CAD build for the part. Positions are in the model's coordinates, mm. Face numbers are marked on the shaded views. A direction names the side the tool comes from. Round coordinates to 2 decimals unless told otherwise and drop trailing zeros. Order: outer loops, then holes, each group sorted by start corner. A loop starts at its lowest first (then second) coordinate and runs counter-clockwise, first axis right, second up.
```python
from build123d import *

# Parameters (mm, degrees)
BOSS_EXTRUDE1_DEPTH = 101.6


with BuildPart() as part:
    # Sketch1 → Boss-Extrude1 (new body)
    with BuildSketch(Plane.XY):
        with BuildLine():
            Line((-101.6, -5178.34108), (-101.6, -5168.81608))
            Line((-101.6, -5168.81608), (-190.441035714, -5168.81608))
            Line((-190.441035714, -5168.81608), (-190.441035714, -5175.16608))
            ThreePointArc((-190.441035714, -5175.16608), (-189.511099745, -5177.41114403), (-187.266035714, -5178.34108))
            Line((-187.266035714, -5178.34108), (-101.6, -5178.34108))
        make_face()
        with BuildLine():
            Line((-38.041035714, -5168.81608), (-47.566035714, -5168.81608))
            Line((-47.566035714, -5168.81608), (-53.408035714, -5168.81608))
            Line((-53.408035714, -5168.81608), (-101.6, -5168.81608))
            Line((-101.6, -5168.81608), (-101.6, -5178.34108))
            Line((-101.6, -5178.34108), (-41.216035714, -5178.34108))
            ThreePointArc((-41.216035714, -5178.34108), (-38.970971684, -5177.41114403), (-38.041035714, -5175.16608))
            Line((-38.041035714, -5175.16608), (-38.041035714, -5168.81608))
        make_face()
        with BuildLine():
            Line((-47.566035714, -5025.94108), (-47.566035714, -5168.81608))
            Line((-47.566035714, -5168.81608), (-38.041035714, -5168.81608))
            Line((-38.041035714, -5168.81608), (-38.041035714, -5029.11608))
            ThreePointArc((-38.041035714, -5029.11608), (-38.970971684, -5026.87101597), (-41.216035714, -5025.94108))
            Line((-41.216035714, -5025.94108), (-47.566035714, -5025.94108))
        make_face()
    extrude(amount=-BOSS_EXTRUDE1_DEPTH)


solid = part.part
```
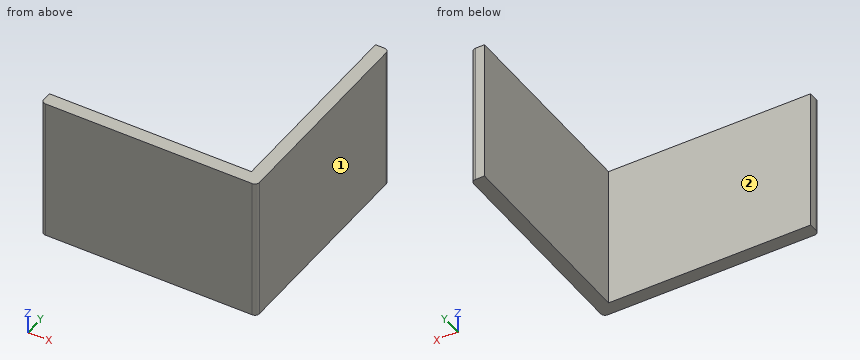
1. Tool access for the marked faces 1 and 2: list every direction of +Z, -Z, +X, -X, +Y, -Y with a clear straight run to the whole face (end or side of a thin tool).
2. Drill centre lines: line 1 (Y direction, x = -164, z = -59); line 2 (X direction, y = -5098.5, z = -32.5). Where is each one in solid material? Low to high.
3. Cut at C-C, the plane y = -5091.5. Write the cut outline in (x, z).
4. Cut at B-B, the plane x = -78. Write the cut outline in (y, z).
5. Pin check, flat tips, straight feed: P1, Ø8, axis at x = -121.5, y = -5162.5, coming from the -Z side; P2, Ø3, axis at x = -155.5, z = -49.5, coming from the +Y side. Stop position of each tip, or through.
6. Cut at A-A, the plane z = -56.5. Write the cut outline in (x, y) (3 decimals), and give its area (3 significant figures).
Outcome:
1. face 1: +Z, -Z, +X, +Y, -Y
1. face 2: +Z, -Z, -X, +Y
2. line 1: y = -5178.34 to -5168.82
2. line 2: x = -47.57 to -38.04
3. outline: (-47.57, -101.6) - (-38.04, -101.6) - (-38.04, 0) - (-47.57, 0) - close
4. outline: (-5178.34, -101.6) - (-5168.82, -101.6) - (-5168.82, 0) - (-5178.34, 0) - close
5. P1: passes through
5. P2: stops at y = -5168.82
6. outline: (-190.441, -5175.166) arc R3.175 ccw to (-187.266, -5178.341) - (-41.216, -5178.341) arc R3.175 ccw to (-38.041, -5175.166) - (-38.041, -5029.116) arc R3.175 ccw to (-41.216, -5025.941) - (-47.566, -5025.941) - (-47.566, -5168.816) - (-190.441, -5168.816) - close
6. area: 2,810 mm2
